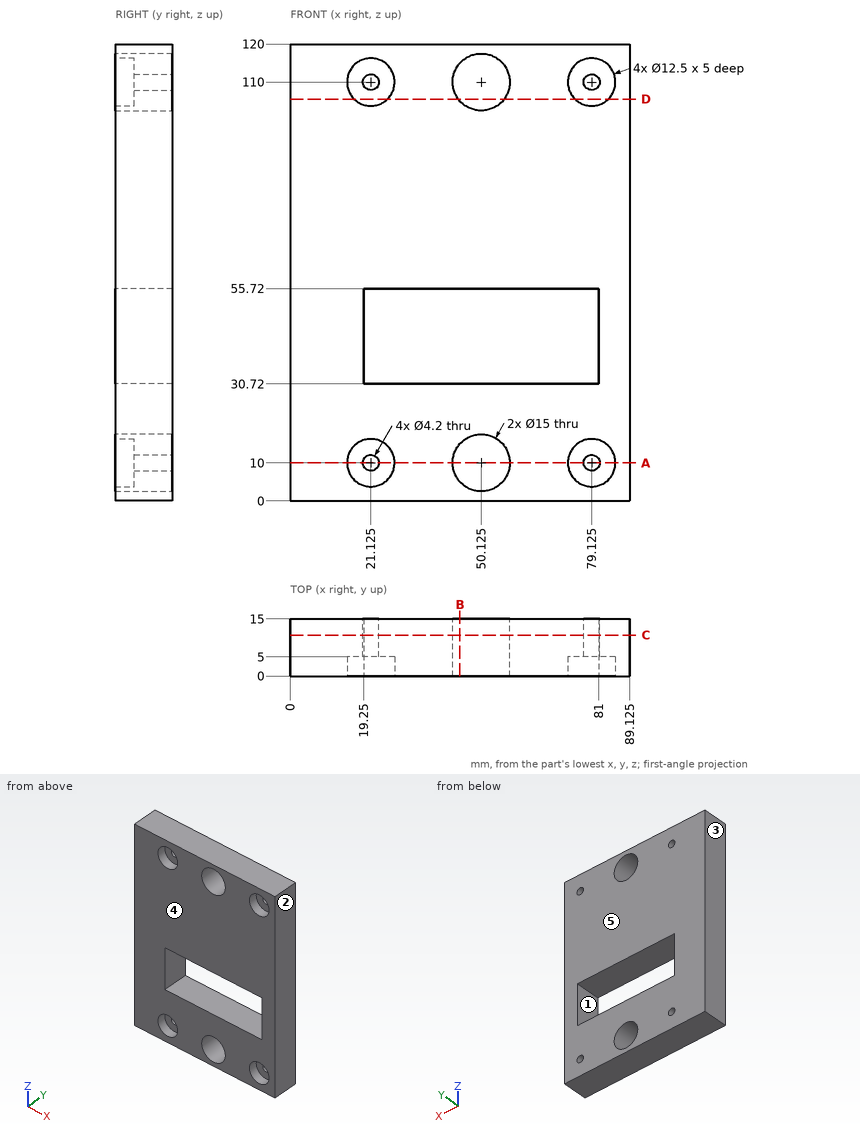
Input: dimensioned drawing with shaded views. Units: mm. Origin: part minimum x, y, z. A direction names the side the tool comes from. Give positions to 0.01 mm unless a question says otherwise; leave off trailing zeros. Loops run counter-clockwise (first coordinate to the right, second up) from the corner with the lowest first, then second, coordinate; pieces in that order, holes last. Notation, with made-up numbers: (0, -29) -> (36, -29) arc R10 cw to (36, -15) -> close; hole circle Ø6 at (-10, 32). An arc over 180 degrees is marked (long way). Use a Markdown table: item, result.
Q1. Section query D-D, the plane z = 105.5. Return the cut outline in (x, y) (3 decimals), plus the area to 3 significant figures.
Entries:
| item | result |
|---|---|
| outline | (0, 0) -> (16.788, 0) -> (16.788, 5) -> (25.462, 5) -> (25.462, 0) -> (44.125, 0) -> (44.125, 15) -> (0, 15) -> close; (56.125, 0) -> (74.788, 0) -> (74.788, 5) -> (83.462, 5) -> (83.462, 0) -> (89.125, 0) -> (89.125, 15) -> (56.125, 15) -> close |
| area | 1,070 mm² |
Q2. Section query A-A, the plane z = 10. Return the cut outline in (x, y) (3 decimals), plus the area to 3 significant figures.
Entries:
| item | result |
|---|---|
| outline | (0, 0) -> (14.875, 0) -> (14.875, 5) -> (19.025, 5) -> (19.025, 15) -> (0, 15) -> close; (23.225, 5) -> (27.375, 5) -> (27.375, 0) -> (42.625, 0) -> (42.625, 15) -> (23.225, 15) -> close; (57.625, 0) -> (72.875, 0) -> (72.875, 5) -> (77.025, 5) -> (77.025, 15) -> (57.625, 15) -> close; (81.225, 5) -> (85.375, 5) -> (85.375, 0) -> (89.125, 0) -> (89.125, 15) -> (81.225, 15) -> close |
| area | 903 mm² |
Q3. Access query for the marked faces 1 and 2. Directions: +Z, -Z, +X, -X, +Y, -Y. A direction counts if a zero-diameter tool reaches every point of the face in a straight line with its end or side. Return the directions, or none.
Entries:
| item | result |
|---|---|
| face 1 | +Y, -Y |
| face 2 | +Z, -Z, +X, +Y, -Y |
Q4. Section query C-C, the plane y = 10.75. Return the cut outline in (x, z) (3 decimals).
Entries:
| item | result |
|---|---|
| outline | (0, 0) -> (89.125, 0) -> (89.125, 120) -> (0, 120) -> close; hole circle Ø4.2 at (21.125, 10); hole circle Ø4.2 at (21.125, 110); hole (19.25, 30.72) -> (81, 30.72) -> (81, 55.72) -> (19.25, 55.72) -> close; hole circle Ø15 at (50.125, 10); hole circle Ø15 at (50.125, 110); hole circle Ø4.2 at (79.125, 10); hole circle Ø4.2 at (79.125, 110) |
Q5. First-contact query: P1, Ø3, axis at y = 3.5, z = 101.5, coming from the -X side; P2, Ø7.5, axis at x = 79.125, z = 110, coming from the -Y side. Flat tips, straight axial feed; report the tip coordinate or a pass-through.
Entries:
| item | result |
|---|---|
| P1 | stops at x = 0 |
| P2 | stops at y = 5 |
Q6. Pull-direction query (Y, two-part tool) for the marked faces 3, 4 and 5; classes: pulls with the +Y half, pulls with the -Y half, needs draft (parallel to the pull), parting line crosses it, or undercut.
Entries:
| item | result |
|---|---|
| face 3 | needs draft |
| face 4 | pulls with the -Y half |
| face 5 | pulls with the +Y half |
Q7. Ray query, probe 1 along X at (y, z) = (10.75, 110) (3 decimals); probe 2 along X at (y, z) = (2.7, 110) (3 decimals); probe 3 along Z at (x, y) = (50.5, 6). Return the intervals inside material, ascending. Write a range as from..to.
Entries:
| item | result |
|---|---|
| probe 1 | x = 0..19.025, 23.225..42.625, 57.625..77.025, 81.225..89.125 |
| probe 2 | x = 0..14.875, 27.375..42.625, 57.625..72.875, 85.375..89.125 |
| probe 3 | z = 0..2.51, 17.49..30.72, 55.72..102.51, 117.49..120 |
Q8. Section query B-B, the plane x = 44.5. Return the cut outline in (y, z).
Entries:
| item | result |
|---|---|
| outline | (0, 0) -> (15, 0) -> (15, 5.04) -> (0, 5.04) -> close; (0, 14.96) -> (15, 14.96) -> (15, 30.72) -> (0, 30.72) -> close; (0, 55.72) -> (15, 55.72) -> (15, 105.04) -> (0, 105.04) -> close; (0, 114.96) -> (15, 114.96) -> (15, 120) -> (0, 120) -> close |
